Part model, mm, in its own coordinate system. Face numbers are marked on the shaded views. A direction names the side the tool comes from. Coordinates: 2 decimals unless noted, no trailing zeros. Write each loop counter-clockwise with the first axis right and the second up, starting at its lowest first coordinate (ties: lowest second). Pieces come first, ordered by that corner, then holes. Notation, with made-up numbers: (-2, 46.25) -> (11, 46.25) arc R20 cw to (11, 79.25) -> close; hole circle Ø6 at (46, 16.25). An arc over 180 degrees is marked (long way). Write item = value, one per line.
from build123d import *

# Parameters (mm, degrees)
F0_W     = 10
F0_H     = 15
F2_DEPTH = 25.4


with BuildPart() as f1:
    # F0 (on Front) → F1 (revolve)
    with BuildSketch(Plane.XZ):
        with BuildLine():
            Line((0, 20), (0, -20))
            ThreePointArc((0, -20), (20, 0), (0, 20))
        make_face()
    revolve(axis=Axis((0, 0, 0), (0, 0, -1)))



with BuildPart() as f1b:
    # F0 (on Front) → F1, piece 2 (revolve)
    with BuildSketch(Plane.XZ):
        with Locations((5, -27.5)):
            Rectangle(F0_W, F0_H)
    revolve(axis=Axis((0, 0, 0), (0, 0, -1)))


with BuildPart() as f1_1:
    add(f1.part)
    # F2 (add): a face of the model
    f2_faces = [f1b.part.faces().sort_by_distance(p)[0] for p in [
        (0, 0, -20),
    ]]

    add(f1b.part)  # F2 merges F1b
    extrude(f2_faces, amount=F2_DEPTH)


solid = f1_1.part
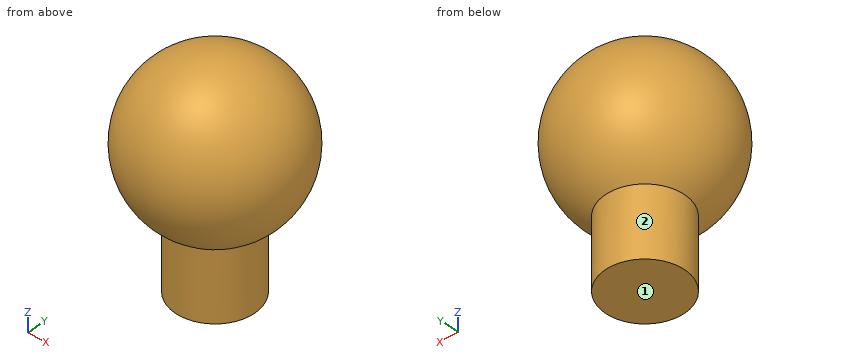
Q1. Probe line 1 (X direction, y = -0.5, z = -29); line 2 (Y direction, x = -3.5, z = 14); line 3 (X direction, y = -13, z = 12). List the from-to ranges inside material, lowest first. Write a range as from..to.
Model answer:
line_1 = -9.99..9.99
line_2 = -13.85..13.85
line_3 = -9.33..9.33
Q2. Which spindle directions (+Z, -Z, +X, -X, +Y, -Y) get a long thin tool onto all of the face, cutting with end or side? Do the marked faces 1 and 2. Say none if no direction does.
Model answer:
face_1 = -Z, +X, -X, +Y, -Y
face_2 = -Z
Q3. Saw through at D-D on y = 14. Give the cut face in (x, z), and give its area (3 significant figures).
Model answer:
outline = circle Ø28.57 at (0, 0)
area = 641 mm²
Q4. Pin check, flat tips, straight feed: pin 1 (6 mm diameter, centred on x = -8, y = 14.5, fed in from -Z); pin 2 (4 mm diameter, centred on x = -14, z = -7.5, fed in from -Y); pin 3 (6 mm diameter, centred on y = -5.5, z = -26, fed in from -X). Stop position of each tip, or through.
Model answer:
pin_1 = -14.7
pin_2 = -14.4
pin_3 = -9.68
Q5. Saw through at A-A on z = 16. Give the cut face in (x, y), and give its area (3 significant figures).
Model answer:
outline = circle Ø24 at (0, 0)
area = 452 mm²
Q6. Saw through at B-B on y = 0. Give the cut face in (x, z).
Model answer:
outline = (-10, -35) -> (10, -35) -> (10, -17.32) arc R20 ccw (long way) to (-10, -17.32) -> close
